The listing builds one solid part. Answer for the finished solid, in the listing's coordinates (mm). Face numbers are marked on the shaded views. A direction names the side the tool comes from. Coordinates: 2 decimals unless noted, no trailing zeros. Order: outer loops, then holes, each group sorted by start corner. A loop starts at its lowest first (then second) coordinate and runs counter-clockwise, first axis right, second up. Notation, with made-up numbers: (21.25, 73) -> (62.25, 73) arc R12 cw to (62.25, 86) -> close; hole circle Ø11 at (1.25, 57.25). An arc over 180 degrees is marked (long way). One line per question, with ' | ' between items.
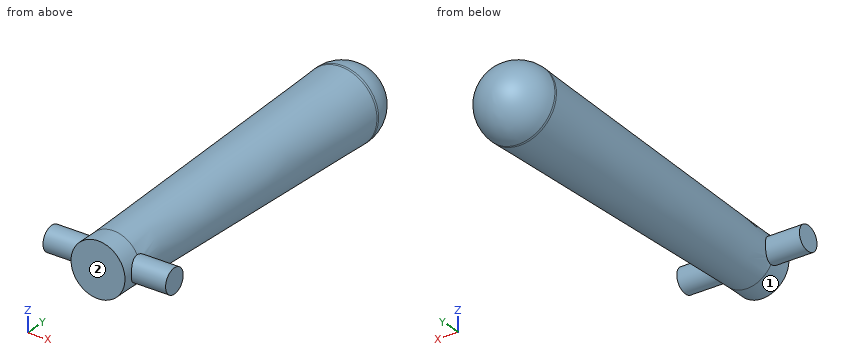
from build123d import *

# Parameters (mm, degrees)
ESQUISSE2_R             = 0.5
BOSS_EXTRU_1_DEPTH      = 2.5
BOSS_EXTRU_1_DEPTH_BACK = 2.5
SCALE1_SCALE            = 0.64015


with BuildPart() as part:
    # Esquisse1 → R_volution1 (revolve)
    with BuildSketch(Plane(origin=(0, 0, 0), x_dir=(0, 0, -1), z_dir=(1, 0, 0))):
        with BuildLine():
            Line((1.49716245, 12.907779617), (1.5, 13))
            ThreePointArc((1.5, 13), (1.060660172, 14.060660172), (0, 14.5))
            Line((0, 14.5), (0, -0.857830241))
            Line((0, -0.857830241), (1.1, -0.857830241))
            Line((1.1, -0.857830241), (1.1, 0))
            Line((1.1, 0), (1.49716245, 12.907779617))
        make_face()
    revolve(axis=Axis((0, 0, 0), (0, 1, 0)))

    # Esquisse2 → Boss.-Extru.1 (add, two sides)
    with BuildSketch(Plane(origin=(0, 0, 0), x_dir=(0, 0, -1), z_dir=(1, 0, 0))) as boss_extru_1_sk:
        Circle(ESQUISSE2_R)
    extrude(amount=BOSS_EXTRU_1_DEPTH)
    extrude(boss_extru_1_sk.sketch, amount=-BOSS_EXTRU_1_DEPTH_BACK)


with BuildPart() as part_1:
    # Scale1: scaled about (0, 7.215672801, 1.5e-08)
    add(part.part.scale(SCALE1_SCALE).moved(Location((0, 2.596559857, 5e-09))))


solid = part_1.part
Item 1: For the marked faces 1 and 2, determine the directions among +Z, -Z, +X, -X, +Y, -Y from which every point of the face is accessible in a straight line to the end or side of a thin tool.
Computed values:
face 1: -Y | face 2: +Z, -Z, +X, -X, -Y
Item 2: Find the intervals of material crossed by L1, parallel to Z at x = 0.55, y = 5.5; L2, parallel to X at y = 2.5, z = -0.6; L3, parallel to X at y = 10.5, z = 0.25, in increasing order.
Computed values:
L1: z = -0.57 to 0.57 | L2: x = -0.37 to 0.37 | L3: x = -0.91 to 0.91
Item 3: Section B-B, the plane y = 11.25 is taken. Give the vertices of the cut face in (x, z), plus the area to 3 significant figures.
Computed values:
outline: circle Ø1.8 at (0, 0) | area: 2.55 mm^2
Item 4: Section A-A, the plane x = 1.1 is taken. Give the vertices of the cut face in (y, z).
Computed values:
outline: circle Ø0.64 at (2.6, 0)
